Job drawing, mm, ordinate dimensions from the low corner. One solid piece. A direction names the side the tool comes from. Give positions to 0.01 mm unless a question says otherwise; leave off trailing zeros. Write each loop counter-clockwise with the first axis right and the second up, starting at its lowest first coordinate (ties: lowest second). Pieces come first, ordered by that corner, then holes. Notation, with made-up numbers: (39.5, 64.5) - (76.5, 64.5) arc R19 ccw to (76.5, 71.5) - close; hole circle Ø1 at (22.5, 49.25). An arc over 180 degrees is marked (long way). Answer as a JSON object with one key per item and string values.
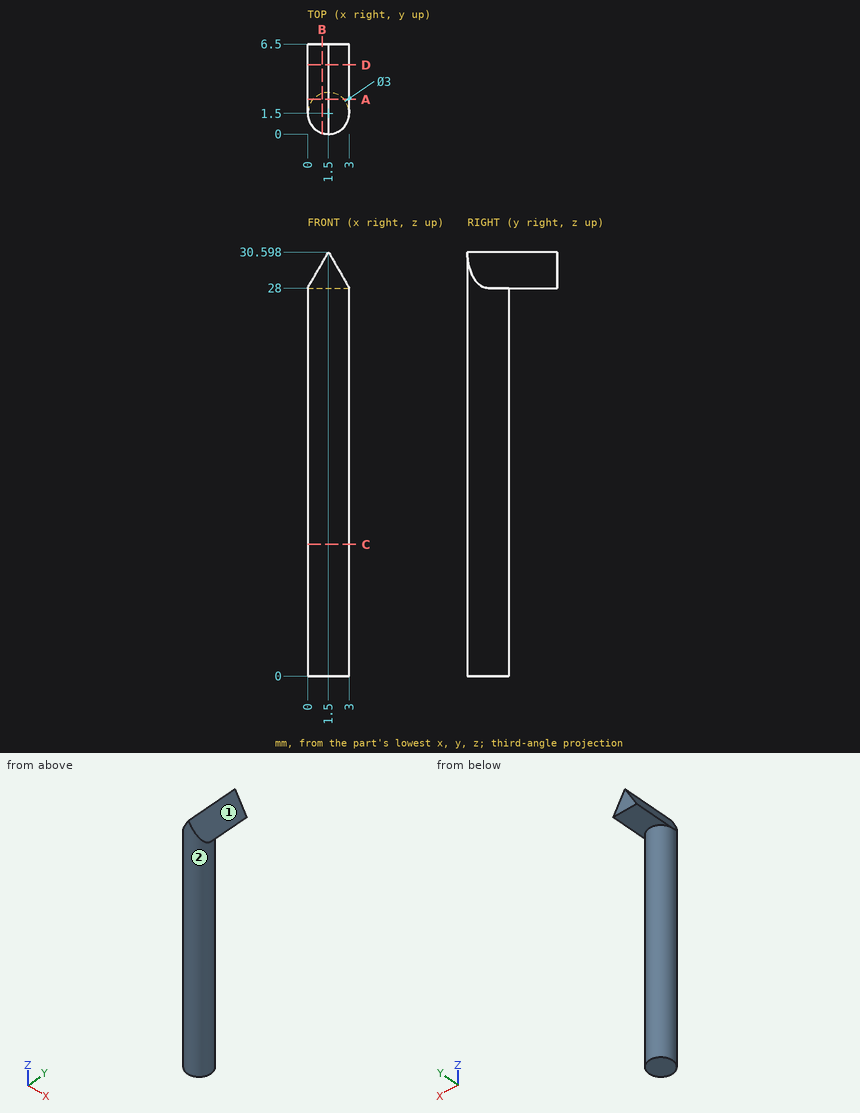
Item 1: Flat gauge pins, fed straight in: P1, Ø2, axis at y = 1, z = 14, coming from the +X side; P2, Ø0.9, axis at x = 1, y = 3.5, coming from the -Z side. Where does each tip first touch, or does it go through?
Entries:
{"P1": "x = 3", "P2": "z = 28"}
Item 2: Cut at D-D (y = 5). Give the cut face in (x, z).
Entries:
{"outline": "(0, 28) - (3, 28) - (1.5, 30.6) - close"}
Item 3: Cut at B-B (x = 1.05). Give the cut face in (y, z), and give its area (3 significant figures).
Entries:
{"outline": "(0.07, 0) - (2.93, 0) - (2.93, 28) - (6.5, 28) - (6.5, 29.82) - (0.07, 29.82) - close", "area": "91.8 mm2"}
Item 4: Probe line 1 (Y direction, x = 1.5, z = 2.5); line 2 (Y direction, x = 2.4, z = 23); line 3 (Z direction, x = 2.35, y = 5.25). List the from-to ranges inside material, lowest first. Write a range as from..to.
Entries:
{"line 1": "0..3", "line 2": "0.3..2.7", "line 3": "28..29.13"}
Item 5: Cut at C-C (z = 9.5). Give the cut face in (x, y).
Entries:
{"outline": "circle Ø3 at (1.5, 1.5)"}
Item 6: Cut at A-A (y = 2.5). Give the cut face in (x, z).
Entries:
{"outline": "(0, 28) - (0.38, 28) - (0.38, 0) - (2.62, 0) - (2.62, 28) - (3, 28) - (1.5, 30.6) - close"}
Item 7: Which spindle directions (+Z, -Z, +X, -X, +Y, -Y) get a long thin tool onto all of the face, cutting with end or side? Do the marked faces 1 and 2. Say none if no direction does.
Entries:
{"face 1": "+Z, +X, +Y, -Y", "face 2": "-Z"}
